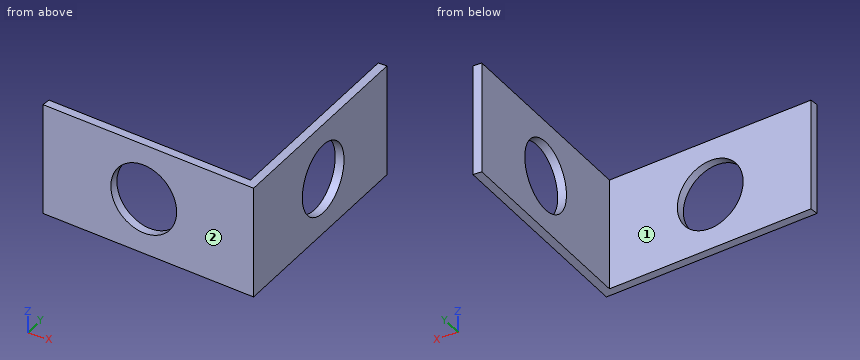
```python
from build123d import *

# Parameters (mm, degrees)
BOSS_EXTRUDE1_DEPTH            = 6.35
F_5_16_0_3125_DIAMETER_HOLE1_D = 7.9375
F_5_16_0_3125_DIAMETER_HOLE2_D = 7.9375


with BuildPart() as part:
    # Sketch1 → Boss-Extrude1 (new body, symmetric)
    with BuildSketch(Plane.XY):
        Polygon((0, 0), (0, 25.4), (-1, 25.4), (-1, 1.091974256), (-25.214234797, 3.225269541), (-25.301995741, 2.229127977), align=None)
    extrude(amount=BOSS_EXTRUDE1_DEPTH, both=True)

    # 5/16 (0.3125) Diameter Hole1 (through all)
    with Locations(Plane(origin=(-1, 13.245987128, 0), x_dir=(0, -1, 0), z_dir=(-1, 0, 0))):
        with Locations((0, 0)):
            Hole(F_5_16_0_3125_DIAMETER_HOLE1_D / 2)

    # 5/16 (0.3125) Diameter Hole2 (through all)
    with Locations(Plane(origin=(-13.107117398, 2.158621899, 0), x_dir=(0.996141565, -0.087760944, 0), z_dir=(0.087760944, 0.996141565, 0))):
        with Locations((0, 0)):
            Hole(F_5_16_0_3125_DIAMETER_HOLE2_D / 2)


solid = part.part
```
Verification items for the finished model (mm, model axes). Face numbers are marked on the shaded views. A direction names the side the tool comes from. Coordinates: 2 decimals unless noted, no trailing zeros. Loops run counter-clockwise (first coordinate to the right, second up) from the corner with the lowest first, then second, coordinate; pieces in that order, holes last. Notation, with made-up numbers: (68, 13.5) - (96, 13.5) arc R13 ccw to (96, 28.5) - close; hole circle Ø1 at (-39, 6.25). An arc over 180 degrees is marked (long way). Put each result on its own line as item: value.
Item 1: Section check D-D (x = -7). Enter the section's corners in (y, z), then the cut area to 3 significant figures.
Conclusion:
outline: (0.62, -6.35) - (1.62, -6.35) - (1.62, 6.35) - (0.62, 6.35) - close
area: 12.7 mm2
Item 2: Section check B-B (y = 16). Enter the section's corners in (x, z).
Conclusion:
outline: (-1, -6.35) - (0, -6.35) - (0, -2.86) - (-1, -2.86) - close; (-1, 2.86) - (0, 2.86) - (0, 6.35) - (-1, 6.35) - close
Item 3: Scan lines: line 1 along X through (y, z) = (17, 5.75); line 2 along Y through (x, z) = (-14, -4.75); line 3 along Y through (x, z) = (-18.25, -5.5). Record each from-to range of solid material in increasing order.
Conclusion:
line 1: x = -1 to 0
line 2: y = 1.23 to 2.24
line 3: y = 1.61 to 2.61
Item 4: Gauge pin test, flat ends, axial feed: pin 1 Ø3 at (x, z) = (-6, -4) entering from +Y; pin 2 Ø4 at (y, z) = (22, 0.5) entering from -X; pin 3 Ø2 at (x, z) = (-15.5, 2) entering from +Y. Record the tip position at first contact, or that the pin passes through.
Conclusion:
pin 1: stops at y = 1.66
pin 2: stops at x = -1
pin 3: stops at y = 2.46
Item 5: Section check C-C (y = 22). Enter the section's corners in (x, z), then the cut area to 3 significant figures.
Conclusion:
outline: (-1, -6.35) - (0, -6.35) - (0, 6.35) - (-1, 6.35) - close
area: 12.7 mm2
Item 6: Section check A-A (z = -0.5). Enter the section's corners in (x, y).
Conclusion:
outline: (-25.3, 2.23) - (-17.12, 1.51) - (-17.03, 2.5) - (-25.21, 3.23) - close; (-9.27, 0.82) - (0, 0) - (0, 9.31) - (-1, 9.31) - (-1, 1.09) - (-9.19, 1.81) - close; (-1, 17.18) - (0, 17.18) - (0, 25.4) - (-1, 25.4) - close
Item 7: Set-up check for the marked faces 1 and 2: record each of +Z, -Z, +X, -X, +Y, -Y from which the full face is reachable in a straight line by a thin tool's end or side.
Conclusion:
face 1: +Z, -Z, +Y
face 2: +Z, -Z, -X, -Y
